Part print with two shaded views. Sizes in mm from the minimum x, y, z corner. A direction names the side the tool comes from. Coordinates: 2 decimals unless noted, no trailing zeros. Loops run counter-clockwise (first coordinate to the right, second up) from the corner with the lowest first, then second, coordinate; pieces in that order, holes last. Notation, with made-up numbers: (-23.5, 55.5) - (-18.5, 55.5) arc R24 ccw to (-18.5, 91.5) - close; hole circle Ø4 at (88, 59). An arc over 180 degrees is marked (long way). Write each question's results on one line, items separated by ' | '. Start each with the question number.
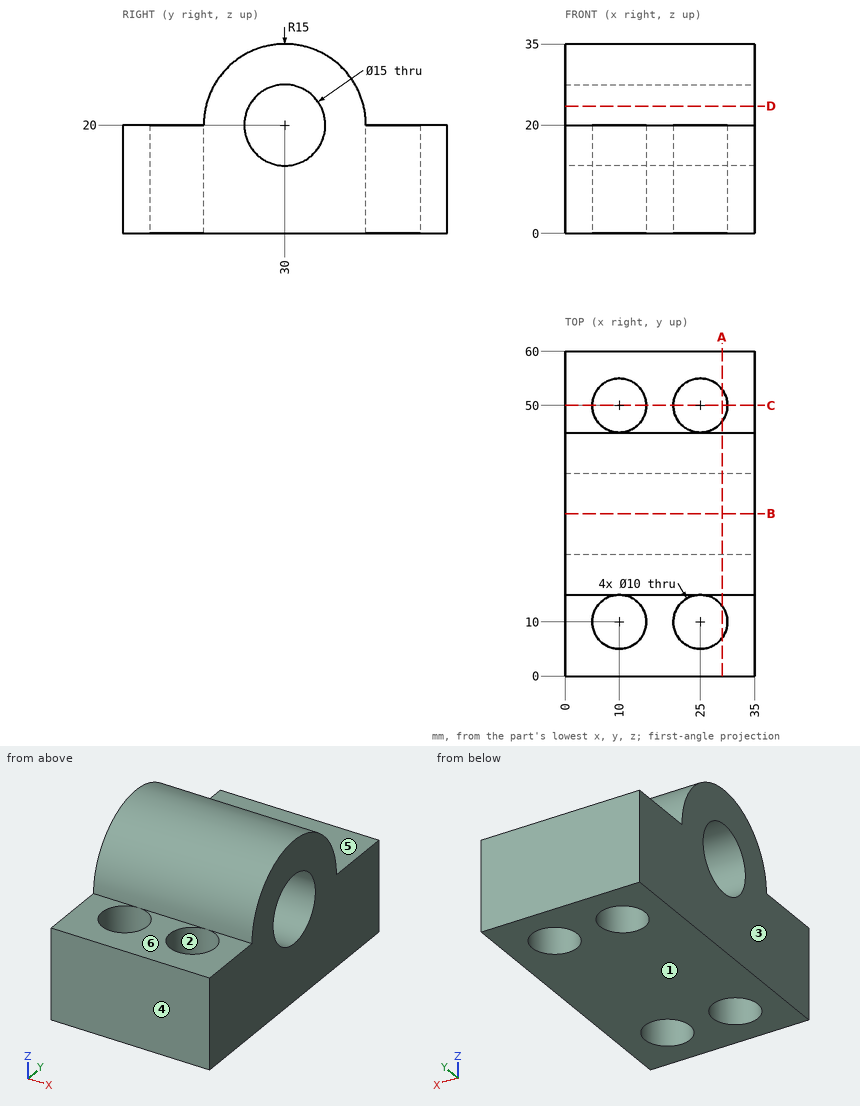
Q1. Pin check, flat tips, straight feed: pin 1 (2 mm diameter, centred on x = 25.5, y = 53, fed in from -Z); pin 2 (7.5 mm diameter, centred on x = 14.5, y = 8, fed in from +Z); pin 3 (4 mm diameter, centred on x = 4.5, z = 29.5, fed in from +Y); pin 4 (13 mm diameter, centred on x = 10, y = 50, fed in from +Z). Stop position of each tip, or through.
Q2. Cut at B-B (y = 30). List the corners of the cut face in (x, z), and give its area (3 significant figures).
Q3. Mould opens along X. For the marked faces 1, 2 and 3 say: +X half, -X half, draft (parallel to the pull), parting line (faces both ways), or undercut.
Q4. Which spindle directions (+Z, -Z, +X, -X, +Y, -Y) get a long thin tool onto all of the face, cutting with end or side? Do the marked faces 4, 5 and 6. Say none if no direction does.
Q5. Cut at D-D (z = 23.5). List the corners of the cut face in (x, y), and give its area (3 significant figures).
Q6. Drill centre lines: L1, parallel to X at y = 10, z = 8; L2, parallel to Y at x = 25, z = 6.5; L3, parallel to Y at x = 27, z = 17. Where is each one in solid material? Low to high. Write a range as from..to.
Q7. Cut at A-A (x = 29). List the corners of the cut face in (y, z), and give its area (3 significant figures).
Q8. Cut at C-C (y = 50). List the corners of the cut face in (x, z).
Check result:
1) pin 1: through | pin 2: z = 20 | pin 3: y = 42.99 | pin 4: z = 26.54
2) outline: (0, 0) - (35, 0) - (35, 12.5) - (0, 12.5) - close; (0, 27.5) - (35, 27.5) - (35, 35) - (0, 35) - close | area: 700 mm²
3) face 1: draft | face 2: undercut | face 3: -X half
4) face 4: +Z, -Z, +X, -X, -Y | face 5: +Z, +X, -X, +Y | face 6: +Z, +X, -X, -Y
5) outline: (0, 15.41) - (35, 15.41) - (35, 23.37) - (0, 23.37) - close; (0, 36.63) - (35, 36.63) - (35, 44.59) - (0, 44.59) - close | area: 557 mm²
6) L1: 0..5, 15..20, 30..35 | L2: 0..5, 15..45, 55..60 | L3: 0..5.42, 14.58..23.13, 36.87..45.42, 54.58..60
7) outline: (0, 0) - (7, 0) - (7, 20) - (0, 20) - close; (13, 0) - (47, 0) - (47, 20) - (45, 20) arc R15 ccw to (15, 20) - (13, 20) - close; (53, 0) - (60, 0) - (60, 20) - (53, 20) - close; hole circle Ø15 at (30, 20) | area: 1,140 mm²
8) outline: (0, 0) - (5, 0) - (5, 20) - (0, 20) - close; (15, 0) - (20, 0) - (20, 20) - (15, 20) - close; (30, 0) - (35, 0) - (35, 20) - (30, 20) - close
